from build123d import *

# Parameters (mm, degrees)
BOSS_EXTRUDE1_DEPTH  = 2
CUT_EXTRUDE8_DEPTH   = 192.01112533
SKETCH3_R            = 2.15
CUT_EXTRUDE9_DEPTH   = 192.01112533
SKETCH8_R            = 2.15
CUT_EXTRUDE11_DEPTH  = 192.01112533
FILLET1_R            = 1
SKETCH17_R           = 18.5
SKETCH17_R_2         = 2.15
CUT_EXTRUDE19_DEPTH  = 10
SKETCH19_R           = 1.65
SKETCH19_W           = 84
SKETCH19_H           = 81
CUT_EXTRUDE21_DEPTH  = 192.01112533
FILLET2_R            = 3
SKETCH20_R           = 1.65
CUT_EXTRUDE22_DEPTH  = 192.01112533
SKETCH21_R           = 1.65
CUT_EXTRUDE23_DEPTH  = 192.01112533
CUT_EXTRUDE24_DEPTH  = 192.01112533
FILLET1_OF_MIRROR1_R = 1


with BuildPart() as part:
    # Sketch1 → Boss-Extrude1 (new body)
    with BuildSketch(Plane(origin=(0, 0, 0), x_dir=(1, 0, 0), z_dir=(0, 1, 0))):
        with BuildLine():
            Line((117.5, -115), (-117.5, -115))
            ThreePointArc((-117.5, -115), (-142.248737342, -104.748737342), (-152.5, -80))
            Line((-152.5, -80), (-152.5, 80))
            ThreePointArc((-152.5, 80), (-142.248737342, 104.748737342), (-117.5, 115))
            Line((-117.5, 115), (117.5, 115))
            ThreePointArc((117.5, 115), (142.248737342, 104.748737342), (152.5, 80))
            Line((152.5, 80), (152.5, -80))
            ThreePointArc((152.5, -80), (142.248737342, -104.748737342), (117.5, -115))
        make_face()
    extrude(amount=-BOSS_EXTRUDE1_DEPTH)

    # Sketch2 → Cut-Extrude8 (cut, through all)
    with BuildSketch(Plane(origin=(0, 0, 0), x_dir=(1, 0, 0), z_dir=(0, 1, 0))):
        Polygon((98, -76.4), (98, -16.4), (111, -16.4), (111, 0.6), (135.5, 0.6), (135.5, -76.4), align=None)
    cut_extrude8 = extrude(amount=-CUT_EXTRUDE8_DEPTH, mode=Mode.SUBTRACT)

    # Sketch3 → Cut-Extrude9 (cut, through all)
    with BuildSketch(Plane(origin=(0, 0, 0), x_dir=(1, 0, 0), z_dir=(0, 1, 0))):
        with Locations(Location((92.2, -65.070175326, 0), (0, 0, 270))):
            Circle(SKETCH3_R)
        with Locations(Location((105.2, -10.6, 0), (0, 0, 270))):
            Circle(SKETCH3_R)
        with Locations(Location((141.935832446, -33.3314455, 0), (0, 0, 270))):
            Circle(SKETCH3_R)
    cut_extrude9 = extrude(amount=-CUT_EXTRUDE9_DEPTH, mode=Mode.SUBTRACT)

    # Sketch8 → Cut-Extrude11 (cut, through all)
    with BuildSketch(Plane(origin=(0, 0, 0), x_dir=(1, 0, 0), z_dir=(0, 1, 0))):
        with Locations(Location((-132.5, 90, 0), (0, 0, 270))):
            Circle(SKETCH8_R)
        with Locations(Location((132.5, 90, 0), (0, 0, 270))):
            Circle(SKETCH8_R)
        with Locations(Location((-132.5, -90, 0), (0, 0, 270))):
            Circle(SKETCH8_R)
        with Locations(Location((132.5, -90, 0), (0, 0, 270))):
            Circle(SKETCH8_R)
    extrude(amount=-CUT_EXTRUDE11_DEPTH, mode=Mode.SUBTRACT)

    # Fillet1
    fillet1_edges = [part.edges().sort_by_distance(p)[0] for p in [
        (135.5, -1, 76.4),
        (98, -1, 76.4),
        (98, -1, 16.4),
        (111, -1, 16.4),
        (111, -1, -0.6),
        (135.5, -1, -0.6),
    ]]
    fillet(fillet1_edges, radius=FILLET1_R)

    # Sketch17 → Cut-Extrude19 (cut)
    with BuildSketch(Plane(origin=(0, 0, 0), x_dir=(1, 0, 0), z_dir=(0, 1, 0))):
        with Locations(Location((100, 84, 0), (0, 0, 270))):
            Circle(SKETCH17_R)
        with Locations(Location((121, 101, 0), (0, 0, 270))):
            Circle(SKETCH17_R_2)
        with Locations(Location((121, 67, 0), (0, 0, 270))):
            Circle(SKETCH17_R_2)
        with Locations(Location((76, 84, 0), (0, 0, 270))):
            Circle(SKETCH17_R_2)
    cut_extrude19 = extrude(amount=-CUT_EXTRUDE19_DEPTH, mode=Mode.SUBTRACT)

    # Sketch19 → Cut-Extrude21 (cut, through all)
    with BuildSketch(Plane(origin=(0, 0, 0), x_dir=(1, 0, 0), z_dir=(0, 1, 0))):
        with Locations(Location((-65, 32.5, 0), (0, 0, 270))):
            Circle(SKETCH19_R)
        with Locations(Location((-65, -4.5, 0), (0, 0, 270))):
            Circle(SKETCH19_R)
        with Locations(Location((65, -4.5, 0), (0, 0, 270))):
            Circle(SKETCH19_R)
        with Locations(Location((65, 32.5, 0), (0, 0, 270))):
            Circle(SKETCH19_R)
        with Locations((0, 14)):
            Rectangle(SKETCH19_W, SKETCH19_H)
    extrude(amount=-CUT_EXTRUDE21_DEPTH, mode=Mode.SUBTRACT)

    # Fillet2
    fillet2_edges = [part.edges().sort_by_distance(p)[0] for p in [
        (42, -1, -54.5),
        (42, -1, 26.5),
        (-42, -1, 26.5),
        (-42, -1, -54.5),
    ]]
    fillet(fillet2_edges, radius=FILLET2_R)

    # Sketch20 → Cut-Extrude22 (cut, through all)
    with BuildSketch(Plane(origin=(0, 0, 0), x_dir=(1, 0, 0), z_dir=(0, 1, 0))):
        with Locations(Location((-137.5, 56.5, 0), (0, 0, 270))):
            Circle(SKETCH20_R)
        with Locations(Location((-101.9, 56.5, 0), (0, 0, 270))):
            Circle(SKETCH20_R)
        with Locations(Location((-137.5, 5.9, 0), (0, 0, 270))):
            Circle(SKETCH20_R)
        with Locations(Location((-101.9, 5.9, 0), (0, 0, 270))):
            Circle(SKETCH20_R)
    extrude(amount=-CUT_EXTRUDE22_DEPTH, mode=Mode.SUBTRACT)

    # Sketch21 → Cut-Extrude23 (cut, through all)
    with BuildSketch(Plane(origin=(0, 0, 0), x_dir=(1, 0, 0), z_dir=(0, 1, 0))):
        with Locations(Location((-80, 49, 0), (0, 0, 270))):
            Circle(SKETCH21_R)
        with Locations(Location((-80, -56, 0), (0, 0, 270))):
            Circle(SKETCH21_R)
        with Locations(Location((0, -81, 0), (0, 0, 270))):
            Circle(SKETCH21_R)
        with Locations(Location((50, -56, 0), (0, 0, 270))):
            Circle(SKETCH21_R)
        with Locations(Location((50, 49, 0), (0, 0, 270))):
            Circle(SKETCH21_R)
    extrude(amount=-CUT_EXTRUDE23_DEPTH, mode=Mode.SUBTRACT)

    # Sketch23 → Cut-Extrude24 (cut, through all)
    with BuildSketch(Plane(origin=(0, 0, 0), x_dir=(1, 0, 0), z_dir=(0, 1, 0))):
        with BuildLine():
            Line((32.5, 105.5), (47.5, 105.5))
            ThreePointArc((47.5, 105.5), (49, 107), (47.5, 108.5))
            Line((47.5, 108.5), (32.5, 108.5))
            ThreePointArc((32.5, 108.5), (31, 107), (32.5, 105.5))
        make_face()
        with BuildLine():
            Line((32.5, 62.5), (47.5, 62.5))
            ThreePointArc((47.5, 62.5), (49, 61), (47.5, 59.5))
            Line((47.5, 59.5), (32.5, 59.5))
            ThreePointArc((32.5, 59.5), (31, 61), (32.5, 62.5))
        make_face()
    cut_extrude24 = extrude(amount=-CUT_EXTRUDE24_DEPTH, mode=Mode.SUBTRACT)

    # Mirror1: Cut-Extrude8, Cut-Extrude9, Cut-Extrude19, Cut-Extrude24 across plane
    add(cut_extrude8.mirror(Plane(origin=(0, 0, 0), x_dir=(0, 0, 1), z_dir=(1, 0, 0))), mode=Mode.SUBTRACT)
    add(cut_extrude9.mirror(Plane(origin=(0, 0, 0), x_dir=(0, 0, 1), z_dir=(1, 0, 0))), mode=Mode.SUBTRACT)
    add(cut_extrude19.mirror(Plane(origin=(0, 0, 0), x_dir=(0, 0, 1), z_dir=(1, 0, 0))), mode=Mode.SUBTRACT)
    add(cut_extrude24.mirror(Plane(origin=(0, 0, 0), x_dir=(0, 0, 1), z_dir=(1, 0, 0))), mode=Mode.SUBTRACT)

    # Fillet1 of Mirror1
    fillet1_of_mirror1_edges = [part.edges().sort_by_distance(p)[0] for p in [
        (-135.5, -1, 76.4),
        (-98, -1, 76.4),
        (-98, -1, 16.4),
        (-111, -1, 16.4),
        (-111, -1, -0.6),
        (-135.5, -1, -0.6),
    ]]
    fillet(fillet1_of_mirror1_edges, radius=FILLET1_OF_MIRROR1_R)


solid = part.part
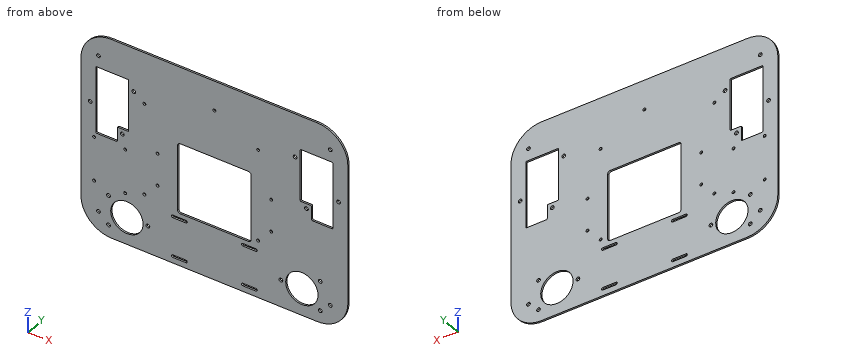
Verification items for the finished model (mm, model axes). Give positions to 0.01 mm unless a question says otherwise; leave off trailing zeros. Loops run counter-clockwise (first coordinate to the right, second up) from the corner with the lowest first, then second, coordinate; pieces in that order, holes last.
1) Thickness scan on line 1 along X through (y, z) = (-0.6, -56.5); line 2 along Z through (x, y) = (-121, -0.45); line 3 along Z through (x, y) = (-27, -1.25). Record the ranges inside material, lowest first.
2) Depth check by flat-ended pin: pin 1 Ø0.6 at (x, y) = (-126.5, -0.5) entering from +Z. Enter the tip coordinate at first touch or a pass-through.
3) Sectioned sample at A-A, the plane z = -11.5. Enter the section's corners in (x, y).
Answers:
1. line 1: x = -152.5 to -139.15, -135.85 to -103.55, -100.25 to 152.5
1. line 2: z = -114.82 to -103.15, -98.85 to -69.15, -64.85 to -0.6, 76.4 to 114.82
1. line 3: z = -115 to -54.5, 26.5 to 115
2. pin 1: stops at z = 113.9
3. outline: (-152.5, -2) - (-42, -2) - (-42, 0) - (-152.5, 0) - close; (42, -2) - (152.5, -2) - (152.5, 0) - (42, 0) - close
